Study the drawing (mm; zero at the part's minimum x, y, z) and answer. Coordinates: 2 decimals unless noted, no trailing zeros. Write each loop counter-clockwise with the first axis right and the second up, starting at its lowest first coordinate (ties: lowest second). Pieces come first, ordered by that corner, then holes. Notation, with made-up numbers: (46.25, 76) -> (104.25, 76) arc R11 ccw to (104.25, 81) -> close; hole circle Ø3 at (-21.5, 60). An arc over 180 degrees is marked (long way). Write item = value, one per line. Start each with the question number.
1) Section C-C (x = 118.7) is taken. Determine the outline of the cut face in (y, z), plus the area to 3 significant figures.
2) Section D-D (y = 9.5) is taken. Count the separate pieces of the cut face and the enclosed holes in it, plus the area to 3 significant figures.
3) Find the intervals of material crossed by line 1 along X through (y, z) = (21.5, 200); line 2 along X through (y, z) = (9, 350), in increasing order. Write a range as from..to.
4) Section A-A (x = 50) is taken. Determine the outline of the cut face in (y, z), plus the area to 3 significant figures.
5) Section B-B (z = 350) is taken. Determine the outline of the cut face in (x, y).
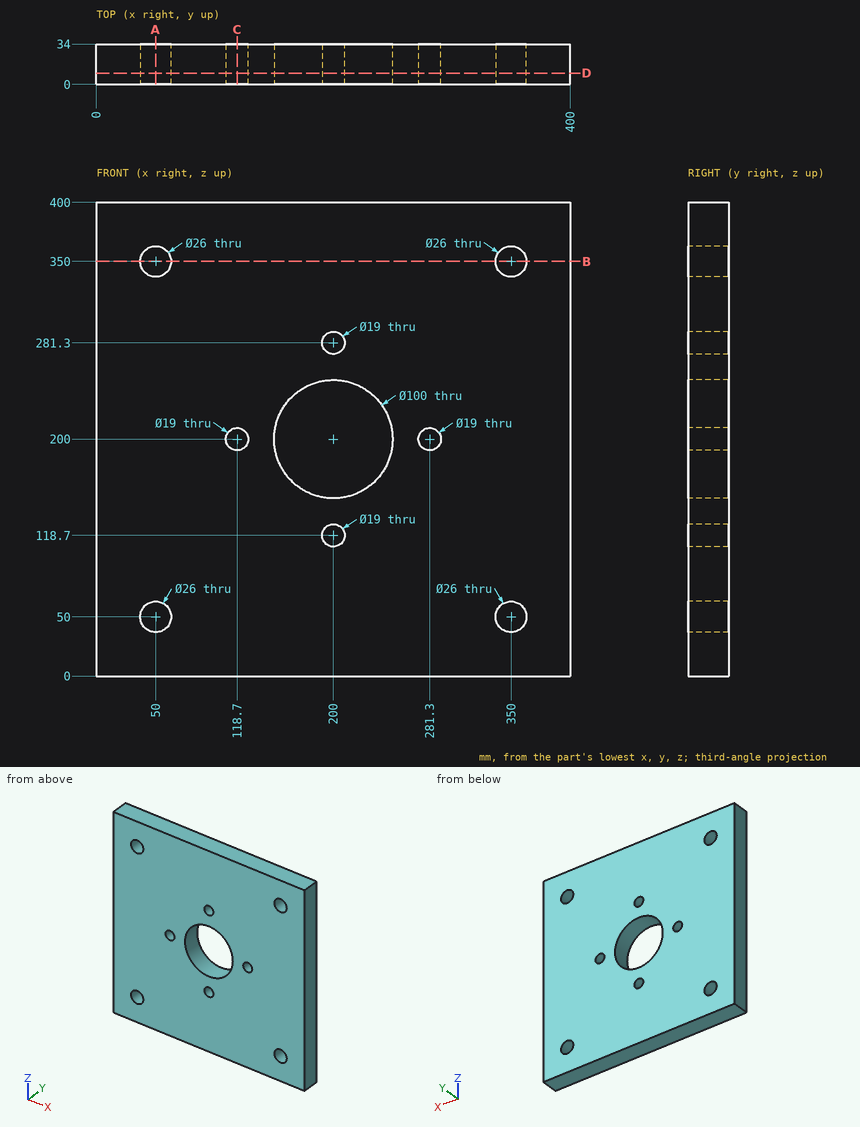
Answer key:
q1.outline = (0, 0) -> (34, 0) -> (34, 190.5) -> (0, 190.5) -> close; (0, 209.5) -> (34, 209.5) -> (34, 400) -> (0, 400) -> close
q1.area = 13,000 mm^2
q2.separate_pieces = 1
q2.enclosed_holes = 9
q2.area = 149,000 mm^2
q3.line_1 = 0..109.2, 128.2..150, 250..271.8, 290.8..400
q3.line_2 = 0..37, 63..337, 363..400
q4.outline = (0, 0) -> (34, 0) -> (34, 37) -> (0, 37) -> close; (0, 63) -> (34, 63) -> (34, 337) -> (0, 337) -> close; (0, 363) -> (34, 363) -> (34, 400) -> (0, 400) -> close
q4.area = 11,800 mm^2
q5.outline = (0, 0) -> (37, 0) -> (37, 34) -> (0, 34) -> close; (63, 0) -> (337, 0) -> (337, 34) -> (63, 34) -> close; (363, 0) -> (400, 0) -> (400, 34) -> (363, 34) -> close
